Design review of the part built by this model. Coordinates are the model's own, in mm. Face numbers are marked on the shaded views. Coordinates: 2 decimals unless noted, no trailing zeros. Loops run counter-clockwise (first coordinate to the right, second up) from the corner with the lowest first, then second, coordinate; pieces in that order, holes last. Notation, with made-up numbers: M -38,-19 L -26,-19 A35 ccw -26,15 Z; hole C 8.25,37 d3. An arc over 180 degrees is marked long. Write item = value, one per line. Start each with the question number.
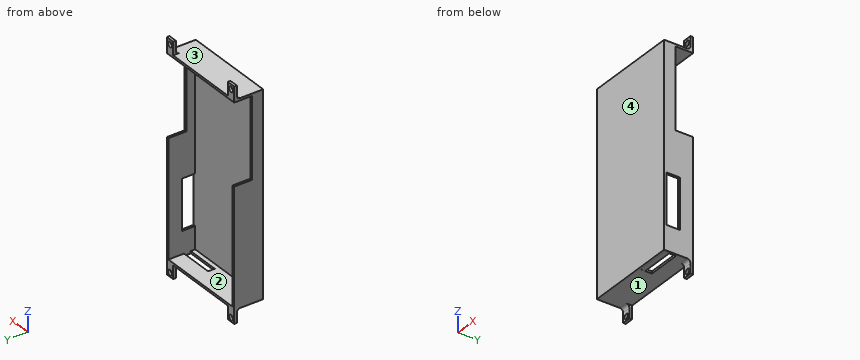
Autodesk Inventor part; units mm, degrees
ref_plane "YZ Plane" through (0, 0, 0) normal (1, 0, 0) x (0, 1, 0)
ref_plane "XZ Plane" through (0, 0, 0) normal (0, 1, 0) x (-1, 0, 0)
ref_plane "XY Plane" through (0, 0, 0) normal (0, 0, 1) x (1, 0, 0)
sketch "Sketch1" plane through (0, 0, 0) normal (0, 1, 0) x (-1, 0, 0)
  line L0 (0, 0) -> (-101.6, 0)
  line L1 (-101.6, 0) -> (-101.6, -223.52)
  line L2 (-101.6, -223.52) -> (0, -223.52)
  line L3 (0, -223.52) -> (0, 0)
  dimension "d0" = 101.6
  dimension "d1" = 223.52
extrude "Extrusion1" add sketch "Sketch1" along normal blind 2.54
sketch "Sketch2" plane through (0, 0, 0) normal (0, -1, 0) x (1, 0, 0)
  line L0 (104.14, 2.54) -> (-2.54, 2.54)
  line L1 (-2.54, 2.54) -> (-2.54, -226.06)
  line L2 (-2.54, -226.06) -> (104.14, -226.06)
  line L3 (104.14, -226.06) -> (104.14, 2.54)
  line L4 (101.6, 0) -> (101.6, -223.52)
  line L5 (0, -223.52) -> (0, 0)
  line L6 (101.6, -223.52) -> (0, -223.52)
  line L7 (0, 0) -> (101.6, 0)
  dimension "d4" = 2.54
  dimension "d5" = 2.54
  dimension "d6" = 2.54
  dimension "d7" = 2.54
extrude "Extrusion2" add sketch "Sketch2" against normal blind 33.02
sketch "Sketch3" plane through (104.14, 0, 2.54) normal (1, 0, 0) x (0, 0, -1)
  line L0 (2.54, 2.54) -> (2.54, 33.02)
  line L1 (2.54, 33.02) -> (93.98, 33.02)
  line L2 (93.98, 33.02) -> (93.98, 12.7)
  line L3 (93.98, 12.7) -> (2.54, 12.7)
  line L4 (2.54, 12.7) -> (2.54, 33.02)
  point P0 (2.54, 0)
  point P1 (2.54, 12.7)
  dimension "d10" = 91.44
  dimension "d11" = 20.32
extrude "Extrusion3" cut sketch "Sketch3" against normal up to surface (106.68 mm away)
sketch "Sketch4" plane through (104.14, 0, -226.06) normal (0, 0, -1) x (-1, 0, 0)
  line L0 (2.54, 2.54) -> (2.54, 12.7)
  line L1 (2.54, 2.54) -> (40.64, 2.54)
  line L2 (40.64, 2.54) -> (40.64, 15.24)
  line L3 (40.64, 15.24) -> (2.54, 15.24)
  line L4 (2.54, 15.24) -> (2.54, 2.54)
  point P0 (104.14, 0)
  point P1 (2.54, 7.62)
  dimension "d14" = 38.1
  dimension "d17" = 12.7
extrude "Extrusion4" cut sketch "Sketch4" against normal up to surface (2.54 mm away)
sketch "Sketch5" plane through (0, 33.02, 0) normal (0, 1, 0) x (1, 0, 0)
  line L0 (104.14, -2.54) -> (-2.54, -2.54)
  line L1 (50.8, -2.54) -> (50.8, -16.5675)
  line L2 (114.0141, 111.76) -> (126.7141, 111.76)
  line L3 (-2.54, -2.54) -> (7.46, -2.54)
  line L4 (7.46, -2.54) -> (7.46, -17.54)
  line L5 (7.46, -17.54) -> (-2.54, -17.54)
  line L6 (-2.54, -17.54) -> (-2.54, -2.54)
  line L7 (-2.54, -2.54) -> (104.14, -2.54)
  line L8 (104.14, -2.54) -> (94.14, -2.54)
  line L9 (94.14, -2.54) -> (94.14, -17.54)
  line L10 (94.14, -17.54) -> (104.14, -17.54)
  line L11 (104.14, -17.54) -> (104.14, -2.54)
  line L12 (104.14, 226.06) -> (-2.54, 226.06)
  line L13 (7.46, 226.06) -> (7.46, 241.06)
  line L14 (7.46, 241.06) -> (-2.54, 241.06)
  line L15 (-2.54, 241.06) -> (-2.54, 226.06)
  line L16 (94.14, 226.06) -> (94.14, 241.06)
  line L17 (104.14, 241.06) -> (104.14, 226.06)
  line L18 (94.14, 241.06) -> (104.14, 241.06)
  point P0 (0, 0)
  dimension "d21" = 10
  dimension "d22" = 15
extrude "Extrusion5" add sketch "Sketch5" against normal blind 3
fillet "Fillet1" radius 4 4 edges at (99.14, 30.02, 2.54) (2.46, 30.02, 2.54) (2.46, 30.02, -226.06) (99.14, 30.02, -226.06)
sketch "Sketch6" plane through (104.14, 0, 2.54) normal (1, 0, 0) x (0, 0, -1)
  point P0 (2.54, 0)
sketch "Sketch7" plane through (104.14, 0, 2.54) normal (1, 0, 0) x (0, 0, -1)
  line L0 (226.06, 2.54) -> (226.06, 15.24)
  line L1 (226.06, 2.54) -> (143.51, 2.54)
  line L2 (143.51, 2.54) -> (143.51, 17.78)
  line L3 (143.51, 17.78) -> (226.06, 17.78)
  line L4 (226.06, 17.78) -> (226.06, 2.54)
  point P0 (2.54, 0)
  dimension "d26" = 82.55
  dimension "d27" = 15.24
extrude "Extrusion6" cut sketch "Sketch7" against normal up to surface (2.54 mm away)
sketch "Sketch8" plane through (0, 33.02, -223.52) normal (0, 0, 1) x (1, 0, 0)
  line L0 (63.5, -30.48) -> (63.5, -17.78)
  line L1 (63.5, -17.78) -> (101.6, -17.78)
  line L2 (101.6, -30.48) -> (101.6, -17.78)
  line L3 (104.14, -30.48) -> (101.6, -30.48)
  line L4 (104.14, -15.24) -> (104.14, -30.48)
  line L5 (104.14, -15.24) -> (101.6, -15.24)
  line L6 (101.6, -15.24) -> (101.6, 0)
  line L7 (0, 0) -> (101.6, 0)
  line L8 (0, -30.48) -> (0, 0)
  line L9 (63.5, -30.48) -> (0, -30.48)
  line L10 (104.14, -30.48) -> (101.6, -30.48)
  line L11 (101.6, -30.48) -> (101.6, -15.24)
  line L12 (101.6, -15.24) -> (104.14, -15.24)
  line L13 (104.14, -15.24) -> (104.14, -30.48)
  point P0 (0, -33.02)
extrude "Extrusion7" add sketch "Sketch8" along normal blind 25.4 contours L11 L5 L4 L3 L2
sketch "Sketch9" plane through (0, 2.54, 0) normal (0, 1, 0) x (1, 0, 0)
  line L0 (63.5, 226.06) -> (63.5, 223.52)
  line L1 (101.6474, 226.008) -> (63.5, 226.008)
  line L2 (63.5, 226.008) -> (63.5, 223.52)
  line L3 (63.5, 223.52) -> (101.6474, 223.52)
  line L4 (101.6474, 223.52) -> (101.6474, 226.008)
  point P0 (0, 0)
extrude "Extrusion8" add sketch "Sketch9" along normal blind 5.08
sketch "Sketch10" plane through (0, 30.02, 0) normal (0, -1, 0) x (1, 0, 0)
  line L0 (-2.54, 17.54) -> (7.46, 17.54)
  line L1 (2.46, 17.54) -> (2.46, 6.54)
  line L2 (7.46, 6.54) -> (-2.54, 6.54)
  line L3 (7.46, 6.54) -> (7.46, 17.54)
  line L4 (7.46, 12.04) -> (-2.54, 12.04)
  line L5 (-2.54, 0) -> (-2.54, 17.54)
  point P0 (0, 0)
  point P1 (2.46, 12.04)
hole "Hole1" at (2.46, 30.02, 12.04) direction (0, 1, 0) diameter 6 depth 3
pattern_linear "Rectangular Pattern1" count 2 spacing 96.68 along (1, 0, 0) count 2 spacing 248.5974 along (0, 0, -1) of "Hole1"
equation "\"d2\" = wallThickness"
equation "\"d4\" = wallThickness"
equation "\"d5\" = wallThickness"
equation "\"d6\" = wallThickness"
equation "\"d7\" = wallThickness"
equation "\"wallThickness\" = 2.54"
properties part number "bms_mount"
Q1. Clearance check with flat-ended pins moving along their axes: P1, Ø1.5, axis at x = 66, z = -44.5, coming from the +Y side; P2, Ø5, axis at x = 96.5, z = -236.5, coming from the -Y side; P3, Ø3, axis at x = -0.5, z = -40, coming from the +Y side; P4, Ø5.5, axis at x = 2.46, z = 12.04, coming from the -Y side. State where each tip first meets the part, or that it passes through.
Q2. To check wall thickness, follow line 1 (Z direction, x = 99.14, y = 32.35); line 2 (X direction, y = 31, z = 12); line 3 (Z direction, x = 18, y = 11.5). State the ranges of each line that lie inside material, in increasing order. Write a range as from..to.
Q3. Add section D-D on z = -170. State the section outline as (x, y) points, plus the area to 3 significant figures.
Q4. Mouldability with a two-part tool opening along Z and no side actions: class the marked faces 1, 2, 3 and 4 as released by +Z, released by -Z, zero draft, split by the parting line, or undercut.
Q5. Add section B-B on z = 12.04. State the section outline as (x, y) points.
Q6. Add section C-C on x = 81.5. State the section outline as (y, z) points, plus the area to 3 significant figures.
Q7. Add section A-A on x = 2.46. State the section outline as (y, z) points.
Values follow:
q1.P1 = 2.54
q1.P2 = 30.02
q1.P3 = 12.7
q1.P4 = through
q2.line_1 = -241.06..-239.56, -233.56..-223.52, 0..9.04, 15.04..17.54
q2.line_2 = -2.54..-0.54, 5.46..7.46, 94.14..96.14, 102.14..104.14
q2.line_3 = -226.06..-223.52, 0..2.54
q3.outline = M -2.54,0 L 104.14,0 L 104.14,2.54 L 0,2.54 L 0,33.02 L -2.54,33.02 Z; M 101.6,17.78 L 104.14,17.78 L 104.14,33.02 L 101.6,33.02 Z
q3.area = 387 mm2
q4.face_1 = released by -Z
q4.face_2 = undercut
q4.face_3 = released by +Z
q4.face_4 = zero draft
q5.outline = M -2.54,30.02 L -0.54,30.02 L -0.54,33.02 L -2.54,33.02 Z; M 5.46,30.02 L 7.46,30.02 L 7.46,33.02 L 5.46,33.02 Z; M 94.14,30.02 L 96.14,30.02 L 96.14,33.02 L 94.14,33.02 Z; M 102.14,30.02 L 104.14,30.02 L 104.14,33.02 L 102.14,33.02 Z
q6.outline = M 0,-226.06 L 2.54,-226.06 L 2.54,-226.01 L 7.62,-226.01 L 7.62,-223.52 L 2.54,-223.52 L 2.54,0 L 33.02,0 L 33.02,2.54 L 0,2.54 Z; M 15.24,-226.06 L 33.02,-226.06 L 33.02,-223.52 L 15.24,-223.52 Z
q6.area = 716 mm2
q7.outline = M 0,-226.06 L 26.02,-226.06 A4 cw 30.02,-230.06 L 30.02,-233.56 L 33.02,-233.56 L 33.02,-223.52 L 2.54,-223.52 L 2.54,0 L 33.02,0 L 33.02,9.04 L 30.02,9.04 L 30.02,6.54 A4 cw 26.02,2.54 L 0,2.54 Z; M 30.02,-241.06 L 33.02,-241.06 L 33.02,-239.56 L 30.02,-239.56 Z; M 30.02,15.04 L 33.02,15.04 L 33.02,17.54 L 30.02,17.54 Z
